Input: part model. Units: mm. Frame: model coordinates. A direction names the side the tool comes from. Coordinates: 2 decimals unless noted, no trailing zeros. Order: outer loops, then holes, each group sorted by start corner. A loop starts at its lowest first (then second) coordinate and runs counter-clockwise, first axis right, second up. Notation, with made-up numbers: (-36.75, 36) - (-10.75, 36) arc R19 ccw to (-10.75, 65) - close; hole circle Ø5 at (-8, -18). An arc over 180 degrees is marked (long way). Answer as CSV lines item,"result". Start each with the question number.
Item 1: First-contact query: pin 1 (4 mm diameter, centred on x = 70.5, y = 1, fed in from +Z); pin 2 (1.3 mm diameter, centred on x = 73, z = 21.5, fed in from -Y); pin 3 (1 mm diameter, centred on x = 17.5, z = 15, fed in from -Y). Flat tips, straight axial feed; report the tip coordinate or a pass-through.
Item 2: Section B-B (x = 21). Output: boundary loops of the cut face in (y, z).
Item 3: Section A-A (x = -129). Output: boundary loops of the cut face in (y, z).
Item 4: Material intervals for line 1 along Y through (x, z) = (-177.75, 0); line 2 along X through (y, z) = (-2.5, -20); line 3 along X through (y, z) = (-24, 0.5), sorted ascending.
Item 5: Draft query along Y for faces 1 (the cylindrical face through (-118.5, 0.1, 17.3)), 2 (the flat face through (-110, 9, -18.1)), 3 (the cylindrical face through (-65.252, 19.961, 10.382)). Return one class per face: +Y half, -Y half, draft (parallel to the pull), parting line (faces both ways), or undercut.
Item 6: Access query for faces 4 (the cylindrical face through (96.34, -6.31, 20.03)), 5 (the flat face through (190, 0, 0)), 6 (the cylindrical face through (-179.86, -13.32, 0.74)), 7 (the cylindrical face through (-181.5, -0.1, 17.3)). Directions: +Z, -Z, +X, -X, +Y, -Y. A direction counts if a zero-diameter tool reaches every point of the face in a straight line with its end or side. Return the directions, or none.
from build123d import *

# Parameters (mm, degrees)
FASE1_SIZE                      = 0.535898385
FASE1_SIZE2                     = 2
FASE1_EDGE_2_SIZE               = 2
FASE1_EDGE_2_SIZE2              = 0.535898385
FASE1_EDGE_3_SIZE               = 2
FASE1_EDGE_3_SIZE2              = 0.535898385
SCHNITT_LINEAR_AUSTRAGEN1_DEPTH = 5.5
M8_GEWINDEBOHRUNG1_D            = 6.8
M8_GEWINDEBOHRUNG1_DEPTH        = 20
M8_GEWINDEBOHRUNG1_TIP          = 2.042926105
FASE2_SIZE                      = 2
FASE2_SIZE2                     = 0.535898385
SCHNITT_LINEAR_AUSTRAGEN2_DEPTH = 1.5


with BuildPart() as part:
    # Skizze1 → Rotation1 (revolve)
    with BuildSketch(Plane.XY, mode=Mode.PRIVATE) as rotation1_sk:
        Polygon((-85, 22.5), (-70, 22.5), (-47, 22.5), (-47, 27.5), (0, 27.5), (0, 0), (-190, 0), (-190, 20), (-110, 20), (-110, 21), (-85, 21), align=None)
    revolve(rotation1_sk.sketch.rotate(Axis((-55.076928245, 0, 0), (1, 0, 0)), 90), axis=Axis((-55.076928245, 0, 0), (1, 0, 0)))  # turned: the seam where the file's is

    # Fase1
    fase1_edges = [part.edges().sort_by_distance(p)[0] for p in [
        (-47, 0, -27.5),
    ]]
    fase1_side = [part.faces().sort_by_distance(p)[0] for p in [
        (-47, 0, -23.277817459),
    ]]
    chamfer(fase1_edges, length=FASE1_SIZE, length2=FASE1_SIZE2, reference=fase1_side[0])

    # Fase1 edge 2
    fase1_edge_2_edges = [part.edges().sort_by_distance(p)[0] for p in [
        (-85, 0, -22.5),
    ]]
    fase1_edge_2_side = [part.faces().sort_by_distance(p)[0] for p in [
        (-66, 0, -22.5),
    ]]
    chamfer(fase1_edge_2_edges, length=FASE1_EDGE_2_SIZE, length2=FASE1_EDGE_2_SIZE2, reference=fase1_edge_2_side[0])

    # Fase1 edge 3
    fase1_edge_3_edges = [part.edges().sort_by_distance(p)[0] for p in [
        (-110, 0, -21),
    ]]
    fase1_edge_3_side = [part.faces().sort_by_distance(p)[0] for p in [
        (-97.5, 0, -21),
    ]]
    chamfer(fase1_edge_3_edges, length=FASE1_EDGE_3_SIZE, length2=FASE1_EDGE_3_SIZE2, reference=fase1_edge_3_side[0])

    # Skizze2 → Schnitt-Linear austragen1 (cut)
    with BuildSketch(Plane.XY.offset(20)):
        with BuildLine():
            Line((-175.5, 6), (-124.5, 6))
            ThreePointArc((-124.5, 6), (-118.5, 0), (-124.5, -6))
            Line((-124.5, -6), (-175.5, -6))
            ThreePointArc((-175.5, -6), (-181.5, 0), (-175.5, 6))
        make_face()
    extrude(amount=-SCHNITT_LINEAR_AUSTRAGEN1_DEPTH, mode=Mode.SUBTRACT)

    # M8 Gewindebohrung1
    with Locations(Plane.ZY.offset(190)):
        with Locations((0, 10), (0, -10)):
            Hole(M8_GEWINDEBOHRUNG1_D / 2, depth=M8_GEWINDEBOHRUNG1_DEPTH)
            with Locations((0, 0, -(M8_GEWINDEBOHRUNG1_DEPTH + M8_GEWINDEBOHRUNG1_TIP / 2))):  # 118° drill point
                Cone(0, M8_GEWINDEBOHRUNG1_D / 2, M8_GEWINDEBOHRUNG1_TIP, mode=Mode.SUBTRACT)

    # Fase2
    fase2_edges = [part.edges().sort_by_distance(p)[0] for p in [
        (-190, 0, -20),
    ]]
    fase2_side = [part.faces().sort_by_distance(p)[0] for p in [
        (-150, 0, -20),
    ]]
    chamfer(fase2_edges, length=FASE2_SIZE, length2=FASE2_SIZE2, reference=fase2_side[0])

    # Skizze8 → Schnitt-Linear austragen2 (cut)
    with BuildSketch(Plane.XY.offset(22.5)):
        with BuildLine():
            Line((-83, 4), (-68, 4))
            ThreePointArc((-68, 4), (-64, 0), (-68, -4))
            Line((-68, -4), (-83, -4))
            Line((-83, -4), (-83, 4))
        make_face()
    extrude(amount=-SCHNITT_LINEAR_AUSTRAGEN2_DEPTH, mode=Mode.SUBTRACT)

    # Spiegeln1: part across plane


with BuildPart() as part_1:
    add(part.part)
    add(part.part.mirror(Plane.ZY))


solid = part_1.part
Determined:
1,pin 1,"stops at z = 21"
1,pin 2,"stops at y = -8.46"
1,pin 3,"stops at y = -23.37"
2,outline,"circle Ø55 at (0, 0)"
3,outline,"(-6, 14.5) - (-6, 19.08) arc R20 ccw (long way) to (6, 19.08) - (6, 14.5) - close"
4,line 1,"y = -20 to -13.4, -6.6 to 6.6, 13.4 to 20"
4,line 2,"x = -110 to 110"
4,line 3,"x = -47 to 47"
5,face 1,"undercut"
5,face 2,"draft"
5,face 3,"parting line"
6,face 4,"+X"
6,face 5,"+Z, -Z, +X, +Y, -Y"
6,face 6,"-X"
6,face 7,"+Z"
